```python
from build123d import *

# Parameters (mm, degrees)
ESBO_O1_W                            = 100
ESBO_O1_H                            = 40
RESSALTO_EXTRUS_O1_DEPTH             = 10
RESSALTO_EXTRUS_O2_DEPTH             = 10
ESBO_O4_W                            = 40
ESBO_O4_H                            = 5.013946539
CORTE_EXTRUS_O1_DEPTH                = 121.933866224
FILETE1_R                            = 8
FURO_DE_DI_METRO_7_0_7_1_D           = 7
FURO_DE_DI_METRO_7_0_7_1_CSINK_D     = 7.05
FURO_DE_DI_METRO_7_0_7_1_CSINK_ANGLE = 90
FILETE2_R                            = 3


with BuildPart() as part:
    # Esboço1 → Ressalto-extrusão1 (new body)
    with BuildSketch(Plane(origin=(0, 0, 0), x_dir=(1, 0, 0), z_dir=(0, 1, 0))):
        with Locations((50, 20)):
            Rectangle(ESBO_O1_W, ESBO_O1_H)
    extrude(amount=RESSALTO_EXTRUS_O1_DEPTH)

    # Esboço3 → Ressalto-extrusão2 (add)
    with BuildSketch(Plane.XY):
        with BuildLine():
            Line((30, 0), (30, 35))
            ThreePointArc((30, 35), (50, 55), (70, 35))
            Line((70, 35), (70, 0))
            Line((70, 0), (30, 0))
        make_face()
    extrude(amount=-RESSALTO_EXTRUS_O2_DEPTH)

    # Esboço4 → Corte-extrusão1 (cut, through all)
    with BuildSketch(Plane.XY):
        with Locations((50, 2.506973269)):
            Rectangle(ESBO_O4_W, ESBO_O4_H)
    extrude(amount=-CORTE_EXTRUS_O1_DEPTH, mode=Mode.SUBTRACT)

    # Esboço6 → Rebaixo para parafuso de cabeça sextavada de M51 (revolve, cut)
    with BuildSketch(Plane(origin=(50, 35, 0), x_dir=(0, -1, 0), z_dir=(1, 0, 0))):
        Polygon((0, 0), (0, 40), (2.75, 40), (2.75, 3.58), (6.12, 3.58), (6.12, 0.025), (6.145, 0), align=None)
    revolve(axis=Axis((50, 35, 6.35), (0, 0, -1)), mode=Mode.SUBTRACT)

    # Filete1
    # the kernel refuses this fillet: 8 mm, written as the material it adds along each edge
    with BuildSketch(Plane(origin=(70, 5.013946539, 0), x_dir=(-1, 0, 0), z_dir=(0, 0, -1))) as filete1_piece_1:
        with BuildLine():
            CenterArc((7.421824892, -8), FILETE1_R, 90, 68.083393909)
            Line((0, -5.013946539), (0, 0))
            Line((0, 0), (7.421824892, 0))
        make_face()
    extrude(amount=40)
    with BuildSketch(Plane(origin=(30, 5.013946539, 0), x_dir=(0, -1, 0), z_dir=(0, 0, -1))) as filete1_piece_2:
        with BuildLine():
            CenterArc((8, -7.421824892), FILETE1_R, 111.916606091, 68.083393909)
            Line((0, -7.421824892), (0, 0))
            Line((0, 0), (5.013946539, 0))
        make_face()
    extrude(amount=40)
    # the kernel refuses this fillet: 8 mm, written as the material it takes off along each edge
    with BuildSketch(Plane(origin=(0, -20, -40), x_dir=(0, 0, 1), z_dir=(0, 1, 0)), Plane(origin=(0, -20, 0), x_dir=(1, 0, 0), z_dir=(0, 1, 0))) as filete1_2_piece_1:
        with BuildLine():
            CenterArc((FILETE1_R, FILETE1_R), FILETE1_R, 180, 90)
            Line((0, FILETE1_R), (0, 0))
            Line((0, 0), (FILETE1_R, 0))
        make_face()
    extrude(amount=50, mode=Mode.SUBTRACT)
    with BuildSketch(Plane(origin=(100, -20, -40), x_dir=(0, 0, 1), z_dir=(0, 1, 0)), Plane(origin=(100, -20, 0), x_dir=(-1, 0, 0), z_dir=(0, 1, 0))) as filete1_2_piece_2:
        with BuildLine():
            CenterArc((FILETE1_R, -FILETE1_R), FILETE1_R, 90, 90)
            Line((0, -FILETE1_R), (0, 0))
            Line((0, 0), (FILETE1_R, 0))
        make_face()
    extrude(amount=50, mode=Mode.SUBTRACT)

    # Furo de diâmetro Ø7.0 (7)1 (through all)
    with Locations(Plane(origin=(0, 10, 0), x_dir=(1, 0, 0), z_dir=(0, 1, 0))):
        with Locations((8, 32), (92, 32)):
            CounterSinkHole(FURO_DE_DI_METRO_7_0_7_1_D / 2, FURO_DE_DI_METRO_7_0_7_1_CSINK_D / 2, counter_sink_angle=FURO_DE_DI_METRO_7_0_7_1_CSINK_ANGLE)

    # Filete2
    filete2_edges = [part.edges().sort_by_distance(p)[0] for p in [
        (81, 10, 0),
        (30, 22.5, -10),
        (70, 22.5, -10),
        (30, 22.5, 0),
        (70, 22.5, 0),
        (50, 55, 0),
        (30, 10, -5),
        (50, 55, -10),
        (70, 10, -5),
        (50, 10, -10),
        (0, 10, -20),
        (50, 10, -40),
        (19, 10, 0),
        (100, 10, -20),
        (97.656854249, 10, -2.343145751),
        (97.656854249, 10, -37.656854249),
        (2.343145751, 10, -2.343145751),
        (2.343145751, 10, -37.656854249),
    ]]
    fillet(filete2_edges, radius=FILETE2_R)


solid = part.part
```
Input: part model. Units: mm. Frame: model coordinates. A direction names the side the tool comes from. Give positions to 0.01 mm unless a question says otherwise; leave off trailing zeros. Order: outer loops, then holes, each group sorted by start corner. A loop starts at its lowest first (then second) coordinate and runs counter-clockwise, first axis right, second up. Notation, with made-up numbers: M 29.25,9.25 L 54.25,9.25 A14 ccw 54.25,14.25 Z; hole C 86.25,80 d2. An arc over 180 degrees is marked long. Return JSON: item names as keys, results as strings.
Item 1: Ray query, probe 1 along X at (y, z) = (7, -32); probe 2 along X at (y, z) = (3, -32); probe 3 along Z at (x, y) = (92, 6.25). Return the intervals inside material, ascending.
Solutions:
{"probe 1": "0 to 4.5, 11.5 to 88.5, 95.5 to 100", "probe 2": "0 to 4.5, 11.5 to 32.11, 67.89 to 88.5, 95.5 to 100", "probe 3": "-40 to -35.5, -28.5 to 0"}
Item 2: Cut plane C-C (x = 14). Return loops of the section in (y, z), then the cut area to 3 significant figures.
Solutions:
{"outline": "M 0,-40 L 7,-40 A3 ccw 10,-37 L 10,-3 A3 ccw 7,0 L 0,0 Z", "area": "396 mm^2"}
Item 3: First-contact query: P1, Ø1.5, axis at x = 38.5, z = -8.5, coming from the +Y side; P2, Ø8, axis at x = 92, z = -32, coming from the +Y side; P3, Ø4, axis at y = 7, z = -4.5, coming from the +X side; P4, Ø13.5, axis at x = 52, y = 38, coming from the +Z side. Flat tips, straight axial feed; report the tip coordinate or a pass-through.
Solutions:
{"P1": "y = 51.54", "P2": "y = 10", "P3": "x = 99.86", "P4": "z = 0"}
Item 4: Cut plane B-B (z = -16.5). Return loops of the section in (x, y).
Solutions:
{"outline": "M 0,0 L 30,0 A8 cw 37.42,5.01 L 62.58,5.01 A8 cw 70,0 L 100,0 L 100,7 A3 ccw 97,10 L 3,10 A3 ccw 0,7 Z"}
Item 5: Cut plane A-A (x = 50). Return loops of the section in (y, z) (3 decimals), then the cut area to 3 significant figures.
Solutions:
{"outline": "M 5.014,-40 L 7,-40 A3 ccw 10,-37 L 10,-13 A3 cw 13,-10 L 32.25,-10 L 32.25,-3.58 L 28.88,-3.58 L 28.88,-0.025 L 28.855,0 L 5.014,0 Z; M 37.75,-10 L 52,-10 A3 ccw 55,-7 L 55,-3 A3 ccw 52,0 L 41.145,0 L 41.12,-0.025 L 41.12,-3.58 L 37.75,-3.58 Z", "area": "566 mm^2"}
Item 6: Access query for faces 1 (the flat face through (50, 5.014, -20)), 2 (the cylindrical face through (69.14, 23.85, -0.9)), 3 (the cylindrical face through (69.1, 23.85, -9.14)), 4 (the cylindrical face through (30.86, 24.15, -0.9)), 5 (the flat face through (30, 24, -5)). Directions: +Z, -Z, +X, -X, +Y, -Y. A direction counts if a zero-diameter tool reaches every point of the face in a straight line with its end or side. Return the directions, or none.
Solutions:
{"face 1": "+Z, -Z, -Y", "face 2": "+Z, +X, +Y", "face 3": "-Z, +X, +Y", "face 4": "+Z, -X, +Y", "face 5": "+Z, -Z, -X, +Y"}
